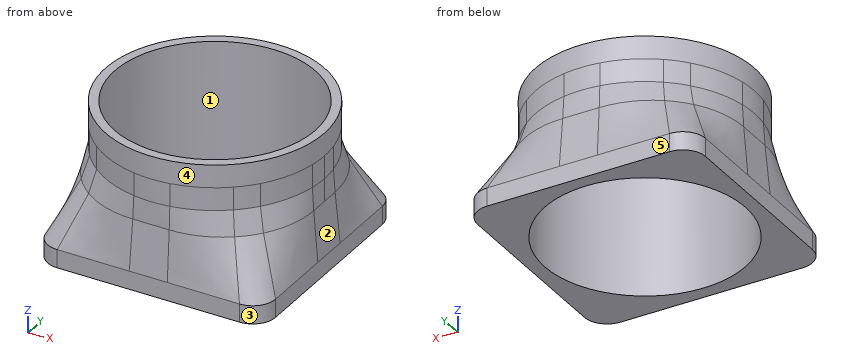
```python
from build123d import *

# Parameters (mm, degrees)
CYLINDER_R     = 22
CYLINDER_DEPTH = 90
SKETCH002_R    = 24
SKETCH003_R    = 24
SKETCH004_R    = 24


with BuildPart() as cylinder:
    # Cylinder → Cylinder (new body)
    with BuildSketch(Plane.XY.offset(-12)):
        Circle(CYLINDER_R)
    extrude(amount=CYLINDER_DEPTH)


with BuildPart() as soporte:
    # Sketch → Loft section 0
    with BuildSketch(Plane.XY):
        with BuildLine():
            Line((-20, 25), (20, 25))
            ThreePointArc((25, 20), (23.535534, 23.535534), (20, 25))
            Line((25, 20), (25, -20))
            ThreePointArc((20, -25), (23.535534, -23.535534), (25, -20))
            Line((20, -25), (-20, -25))
            ThreePointArc((-25, -20), (-23.535534, -23.535534), (-20, -25))
            Line((-25, -20), (-25, 20))
            ThreePointArc((-20, 25), (-23.535534, 23.535534), (-25, 20))
        make_face()
    # Sketch005 → Loft section 1
    with BuildSketch(Plane.XY.offset(4)):
        with BuildLine():
            Line((-20, 25), (20, 25))
            ThreePointArc((25, 20), (23.535534, 23.535534), (20, 25))
            Line((25, 20), (25, -20))
            ThreePointArc((20, -25), (23.535534, -23.535534), (25, -20))
            Line((20, -25), (-20, -25))
            ThreePointArc((-25, -20), (-23.535534, -23.535534), (-20, -25))
            Line((-25, -20), (-25, 20))
            ThreePointArc((-20, 25), (-23.535534, 23.535534), (-25, 20))
        make_face()
    # Sketch006 → Loft section 2
    with BuildSketch(Plane.XY.offset(15)):
        with BuildLine():
            Line((-4, 24), (4, 24))
            ThreePointArc((24, 4), (18.142136, 18.142136), (4, 24))
            Line((24, 4), (24, -4))
            ThreePointArc((4, -24), (18.142136, -18.142136), (24, -4))
            Line((4, -24), (-4, -24))
            ThreePointArc((-24, -4), (-18.142136, -18.142136), (-4, -24))
            Line((-24, -4), (-24, 4))
            ThreePointArc((-4, 24), (-18.142136, 18.142136), (-24, 4))
        make_face()
    # Sketch002 → Loft section 3
    with BuildSketch(Plane.XY.offset(20)):
        Circle(SKETCH002_R)
    # Sketch003 → Loft section 4
    with BuildSketch(Plane.XY.offset(25)):
        with Locations((-0.000114, 0.003714)):
            Circle(SKETCH003_R)
    # Sketch004 → Loft section 5
    with BuildSketch(Plane.XY.offset(30)):
        with Locations((-0.000114, 0.003714)):
            Circle(SKETCH004_R)
    loft(ruled=True)

    # Cut: cut Cylinder
    add(cylinder.part, mode=Mode.SUBTRACT)


solid = soporte.part
```
Input: part model. Units: mm. Frame: model coordinates. Face numbers are marked on the shaded views. A direction names the side the tool comes from. Coordinates: 2 decimals unless noted, no trailing zeros. Loops run counter-clockwise (first coordinate to the right, second up) from the corner with the lowest first, then second, coordinate; pieces in that order, holes last. Notation, with made-up numbers: (-0.5, -26) - (43.5, -26) arc R13 ccw to (43.5, -7) - close; hole circle Ø2 at (52.5, -34). An arc over 180 degrees is marked (long way). Answer in a Markdown table with one row per item.
(1) Cut plane A-A on z = 2. Output: boundary loops of the cut face in (x, y).
Model answer:
| item | result |
|---|---|
| outline | (-25, -20) arc R5 ccw to (-20, -25) - (20, -25) arc R5 ccw to (25, -20) - (25, 20) arc R5 ccw to (20, 25) - (-20, 25) arc R5 ccw to (-25, 20) - close; hole circle Ø44 at (0, 0) |
(2) Material intervals for L1, parallel to Y at x = 0, z = 3.5; L2, parallel to Y at x = 0, z = 16; L3, parallel to X at y = -19.5, z = 27, sorted ascending. Write a range as from..to.
Model answer:
| item | result |
|---|---|
| L1 | y = -25..-22, 22..25 |
| L2 | y = -24..-22, 22..24 |
| L3 | x = -13.99..-10.19, 10.19..13.99 |
(3) Set-up query: the marked faces 4 and 5. Return all of +Z, -Z, +X, -X, +Y, -Y with unobstructed straight access to the full face (end or side cutting, diameter ignored); none if empty.
Model answer:
| item | result |
|---|---|
| face 4 | +Z |
| face 5 | +Z, -Z, +X, -X, +Y |
(4) Mould query, pull axis Y, two halves, no side actions, for the marked faces 1, 2 and 3. Classes: pulls with the +Y half, pulls with the -Y half, needs draft (parallel to the pull), parting line crosses it, or undercut.
Model answer:
| item | result |
|---|---|
| face 1 | undercut |
| face 2 | needs draft |
| face 3 | pulls with the -Y half |
(5) Pin query (flat end, axial travel): P1, Ø10, axis at x = -18, z = 24.5, coming from the +Y side; P2, Ø1.5, axis at x = -0.5, z = 15.5, coming from the +Y side; P3, Ø3, axis at x = -20, y = 19.5, coming from the +Z side. Return the tip coordinate at first contact, or that it passes through.
Model answer:
| item | result |
|---|---|
| P1 | stops at y = 20.18 |
| P2 | stops at y = 24.02 |
| P3 | stops at z = 13.88 |
